```python
from build123d import *

# Parameters (mm, degrees)
SKETCH1_R           = 2.5
BOSS_EXTRUDE1_DEPTH = 1


with BuildPart() as part:
    # Sketch1 → Boss-Extrude1 (new body)
    with BuildSketch(Plane(origin=(0, 0, 0), x_dir=(1, 0, 0), z_dir=(0, 1, 0))):
        Polygon((-102.5, 115), (-97.5, 115), (-97.5, 139), (97.5, 139), (97.5, 115), (102.5, 115), (102.5, 110), (126.5, 110), (126.5, -110), (102.5, -110), (102.5, -115), (97.5, -115), (97.5, -139), (-97.5, -139), (-97.5, -115), (-102.5, -115), (-102.5, -110), (-126.5, -110), (-126.5, 110), (-102.5, 110), align=None)
        with Locations(Location((-114.5, -50, 0), (0, 0, 270))):
            Circle(SKETCH1_R, mode=Mode.SUBTRACT)
        with Locations(Location((-114.5, 50, 0), (0, 0, 270))):
            Circle(SKETCH1_R, mode=Mode.SUBTRACT)
        with Locations(Location((-50, 127, 0), (0, 0, 270))):
            Circle(SKETCH1_R, mode=Mode.SUBTRACT)
        with Locations(Location((50, 127, 0), (0, 0, 270))):
            Circle(SKETCH1_R, mode=Mode.SUBTRACT)
        with Locations(Location((114.5, 50, 0), (0, 0, 270))):
            Circle(SKETCH1_R, mode=Mode.SUBTRACT)
        with Locations(Location((114.5, -50, 0), (0, 0, 270))):
            Circle(SKETCH1_R, mode=Mode.SUBTRACT)
        with Locations(Location((50, -127, 0), (0, 0, 270))):
            Circle(SKETCH1_R, mode=Mode.SUBTRACT)
        with Locations(Location((-50, -127, 0), (0, 0, 270))):
            Circle(SKETCH1_R, mode=Mode.SUBTRACT)
    extrude(amount=BOSS_EXTRUDE1_DEPTH)


solid = part.part
```
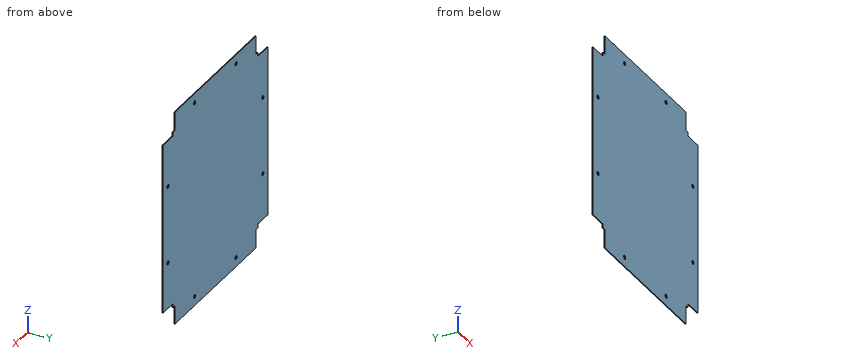
Input: part model. Units: mm. Frame: model coordinates. Give positions to 0.01 mm unless a question says otherwise; leave off trailing zeros. Use a Markdown table: item, result.
(1) Line query: line 1 (X direction, y = 0.2, z = -50); line 2 (X direction, y = 0.65, z = 127); line 3 (X direction, y = 0.5, z = 111). Output: solid intervals per line, ascending. Write a range as from..to.
Computed values:
| item | result |
|---|---|
| line 1 | x = -126.5..-117, -112..112, 117..126.5 |
| line 2 | x = -97.5..-52.5, -47.5..47.5, 52.5..97.5 |
| line 3 | x = -102.5..102.5 |
(2) Pin query (flat end, axial travel): pin 1 (4 mm diameter, centred on x = -50, z = -127, fed in from +Y); pin 2 (0.5 mm diameter, centred on x = -100.5, y = 0.5, fed in from -Z). Return the tip coordinate at first contact, or that it passes through.
Computed values:
| item | result |
|---|---|
| pin 1 | passes through |
| pin 2 | stops at z = -115 |
(3) Section query A-A (y = 0.8). State how many separate pieces and enclosed holes the cut face has, then the cut area to 3 significant figures.
Computed values:
| item | result |
|---|---|
| separate pieces | 1 |
| enclosed holes | 8 |
| area | 66,900 mm2 |
